from build123d import *

# Parameters (mm, degrees)
SKETCH1_R                        = 48
SKETCH1_R_2                      = 8
EX_CARRIER_FRONT_PLATE_4MM_DEPTH = 3
SKETCH2_R                        = 6
CUT_PIN_HOLE_12_DEPTH            = 69.14690015
PAT_PIN_HOLES_3X120_COUNT        = 3
CUT_EXTRUDE1_DEPTH               = 1
SKETCH4_W                        = 10
SKETCH4_H                        = 18
BOSS_EXTRUDE1_DEPTH              = 19
SKETCH5_R                        = 2.1
CUT_EXTRUDE3_DEPTH               = 12
CIRPATTERN1_COUNT                = 3
CIRPATTERN2_COUNT                = 3
SKETCH7_W                        = 4.5
SKETCH7_H                        = 8
CUT_MB6_TAB_GROOVE_6W_M27_DEPTH  = 3


with BuildPart() as part:
    # Sketch1 → EX_Carrier_Front_Plate_4mm (new, symmetric)
    with BuildSketch(Plane.XY):
        Circle(SKETCH1_R)
        Circle(SKETCH1_R_2, mode=Mode.SUBTRACT)
    extrude(amount=EX_CARRIER_FRONT_PLATE_4MM_DEPTH, both=True)

    # Sketch2 → CUT_Pin_Hole__12 (cut, symmetric)
    with BuildSketch(Plane.XY.offset(3)):
        with Locations((0, 33.75)):
            Circle(SKETCH2_R)
    cut_pin_hole_12 = extrude(amount=CUT_PIN_HOLE_12_DEPTH, both=True, mode=Mode.SUBTRACT)

    # PAT_Pin_Holes_3x120: CUT_Pin_Hole__12 ×3 about axis
    pat_pin_holes_3x120_axis = Axis((0, 0, 0), (0, 0, 1))
    for i in range(1, PAT_PIN_HOLES_3X120_COUNT):
        add(cut_pin_hole_12.rotate(pat_pin_holes_3x120_axis, i * 360 / PAT_PIN_HOLES_3X120_COUNT), mode=Mode.SUBTRACT)

    # Sketch3 → Cut-Extrude1 (cut, symmetric)
    with BuildSketch(Plane(origin=(0, 0, 0), x_dir=(0, 0, -1), z_dir=(1, 0, 0))):
        Polygon((-0.476916813, 48), (-3, 44.300014389), (-3, 48), align=None)
    extrude(amount=CUT_EXTRUDE1_DEPTH, both=True, mode=Mode.SUBTRACT)

    # Sketch4 → Boss-Extrude1 (add)
    with BuildSketch(Plane.XY):
        with Locations((0, -33.75)):
            Rectangle(SKETCH4_W, SKETCH4_H)
    boss_extrude1 = extrude(amount=BOSS_EXTRUDE1_DEPTH)

    # Sketch5 → Cut-Extrude3 (cut)
    with BuildSketch(Plane.XY.offset(19)):
        with Locations((0, -33.75)):
            Circle(SKETCH5_R)
    cut_extrude3 = extrude(amount=-CUT_EXTRUDE3_DEPTH, mode=Mode.SUBTRACT)

    # CirPattern1: Boss-Extrude1 ×3 about axis
    cirpattern1_axis = Axis((0, 0, 0), (0, 0, 1))
    for i in range(1, CIRPATTERN1_COUNT):
        add(boss_extrude1.rotate(cirpattern1_axis, i * 360 / CIRPATTERN1_COUNT))

    # CirPattern2: Cut-Extrude3 ×3 about axis
    cirpattern2_axis = Axis((0, 0, 0), (0, 0, 1))
    for i in range(1, CIRPATTERN2_COUNT):
        add(cut_extrude3.rotate(cirpattern2_axis, i * 360 / CIRPATTERN2_COUNT), mode=Mode.SUBTRACT)

    # Sketch6 → Revolve1 (revolve)
    with BuildSketch(Plane(origin=(0, 0, 0), x_dir=(0, 0, -1), z_dir=(1, 0, 0)), mode=Mode.PRIVATE) as revolve1_sk:
        Polygon((2, 0), (2, 18), (6, 18), (6, 15), (58, 15), (58, 14), (65, 14), (65, 12.5), (105, 12.5), (105, 0), align=None)
    revolve(revolve1_sk.sketch.rotate(Axis((0, 0, 4), (0, 0, -1)), 90), axis=Axis((0, 0, 4), (0, 0, -1)))

    # Sketch7 → CUT_MB6_Tab_Groove_6w_M27 (cut, symmetric)
    with BuildSketch(Plane(origin=(0, 0, 0), x_dir=(1, 0, 0), z_dir=(0, 1, 0))):
        with Locations((14.25, 54)):
            Rectangle(SKETCH7_W, SKETCH7_H)
    extrude(amount=CUT_MB6_TAB_GROOVE_6W_M27_DEPTH, both=True, mode=Mode.SUBTRACT)


solid = part.part
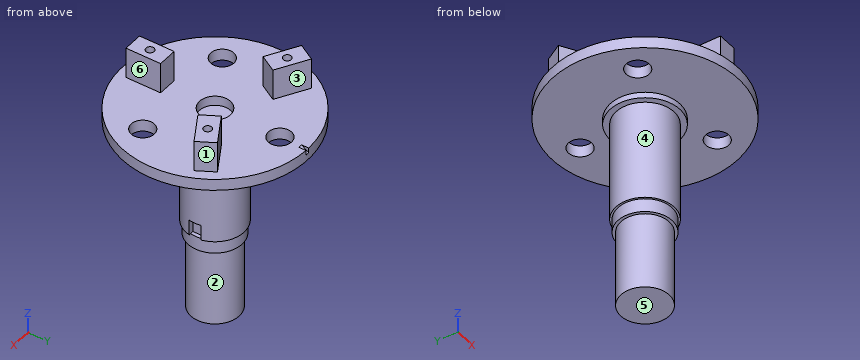
The model under review builds one solid part; all positions refer to its coordinate system, in mm. Face numbers are marked on the shaded views. A direction names the side the tool comes from. Give positions to 0.01 mm unless a question says otherwise; leave off trailing zeros. Order: outer loops, then holes, each group sorted by start corner. A loop starts at its lowest first (then second) coordinate and runs counter-clockwise, first axis right, second up. Notation, with made-up numbers: M 54.5,-28.5 L 98.5,-28.5 A14 cw 98.5,-22.5 Z; hole C 83,1 d4. An arc over 180 degrees is marked long. Answer in a Markdown table with one row per item. Add a question column.
1. For pin 1 Ø5 at (y, z) = (-5, -12) entering from +X; pin 2 Ø2.5 at (x, y) = (-29.23, 16.88) entering from +Z; pin 3 Ø6 at (x, y) = (31, -30) entering from +Z; pin 4 Ø2.5 at (x, y) = (13, 0) entering from -Z, all flat-tipped, find the tip position at first contact; note any pin that passes through.
2. Add section B-B on z = -10.5. State the section outline as (x, y) points.
3. Add section C-C on y = 0. State the section outline as (x, z) points, plus the area to 3 significant figures.
4. Mouldability with a two-part tool opening along X and no side actions: class the marked faces 1, 2 and 3 as released by +X, released by -X, zero draft, split by the parting line, or undercut.
5. Add section D-D on z = -83.5. State the section outline as (x, y) points.
6. To check wall thickness, follow line 1 along Y through (x, z) = (0, 1.35); line 2 along Y through (x, z) = (0, 14.25); line 3 along Z through (x, y) = (-10, -5.5). State the ranges of each line that lie inside material, in increasing order.
7. Add section A-A on y = 38. State the section outline as (x, z) points, plus the area to 3 significant figures.
8. Machinability: for the marked faces 4, 5 and 6, which of the approach directions +Z, -Z, +X, -X, +Y, -Y give a long, thin tool a straight path to every point of the face, cutting with its end or side? Answer none if there is none.
The answers:
| question | item | result |
|---|---|---|
| 1 | pin 1 | x = 14.79 |
| 1 | pin 2 | z = 7 |
| 1 | pin 3 | z = 3 |
| 1 | pin 4 | z = -105 |
| 2 | outline | C 0,0 d30 |
| 3 | outline | M -48,-3 L -18,-3 L -18,-6 L -15,-6 L -15,-58 L -14,-58 L -14,-65 L -12.5,-65 L -12.5,-105 L 12.5,-105 L 12.5,-65 L 14,-65 L 14,-58 L 12,-58 L 12,-50 L 15,-50 L 15,-6 L 18,-6 L 18,-3 L 48,-3 L 48,3 L 8,3 L 8,-2 L -8,-2 L -8,3 L -48,3 Z |
| 3 | area | 3,340 mm2 |
| 4 | face 1 | released by +X |
| 4 | face 2 | split by the parting line |
| 4 | face 3 | undercut |
| 5 | outline | C 0,0 d25 |
| 6 | line 1 | -48 to -8, 8 to 27.75, 39.75 to 46.72 |
| 6 | line 2 | -42.75 to -35.85, -31.65 to -24.75 |
| 6 | line 3 | -105 to 3 |
| 7 | outline | M -29.33,-3 L -4.24,-3 L -4.24,3 L -29.33,3 Z; M 4.24,-3 L 29.33,-3 L 29.33,3 L 4.24,3 Z |
| 7 | area | 301 mm2 |
| 8 | face 4 | -Z |
| 8 | face 5 | -Z, +X, -X, +Y, -Y |
| 8 | face 6 | +Z, +X, +Y, -Y |
